Input: part model. Units: mm. Frame: model coordinates. Face numbers are marked on the shaded views. A direction names the side the tool comes from. Round coordinates to 2 decimals unless told otherwise and drop trailing zeros. Write each loop counter-clockwise with the first axis right and the second up, starting at its lowest first coordinate (ties: lowest second). Pieces come first, ordered by that corner, then holes. Notation, with made-up numbers: (56, -24) -> (60, -24) arc R15 cw to (60, -8) -> close; hole circle Ø7 at (66.5, -17.75). An arc over 180 degrees is marked (long way). Write item = value, one per line.
```python
from build123d import *

# Parameters (mm, degrees)
F0_W     = 58.7502
F0_H     = 43.18
F1_DEPTH = 22.225
F2_T     = -1.5875
F3_W     = 14.2875
F3_H     = 17.4625
F4_DEPTH = 3.175
F6_DEPTH = 0.79375
F7_R     = 2.54
F8_DEPTH = 6.35


with BuildPart() as f1:
    # F0 (on Front) → F1 (new body)
    with BuildSketch(Plane.XZ):
        with Locations((-10.3959683329, -10.1375534884)):
            Rectangle(F0_W, F0_H)
    extrude(amount=F1_DEPTH)

    # F2
    f2_openings = [f1.faces().sort_by_distance(p)[0] for p in [
        (-10.395968, -11.1125, 11.452447),
    ]]
    offset(amount=F2_T, openings=f2_openings)

    # F3 (on face) → F4 (cut)
    with BuildSketch(Plane.XZ.offset(22.225)):
        with BuildLine():
            Line((17.1960732201, 11.4524465116), (-11.3789267799, 11.4524465116))
            Line((-11.3789267799, 11.4524465116), (-11.3789267799, -3.0465692528))
            ThreePointArc((-11.3789267799, -3.0465692528), (2.9085732201, -13.7111715641), (17.1960732201, -3.0465692528))
            Line((17.1960732201, -3.0465692528), (17.1960732201, 11.4524465116))
        make_face()
        with Locations((-28.0476767799, -1.7169438296)):
            Rectangle(F3_W, F3_H)
        with BuildLine():
            Line((-13.4438804602, -15.5461690363), (-27.7313804602, -15.5461690363))
            ThreePointArc((-27.7313804602, -15.5461690363), (-34.0813804602, -21.8961690363), (-27.7313804602, -28.2461690363))
            Line((-27.7313804602, -28.2461690363), (-13.4438804602, -28.2461690363))
            Line((-13.4438804602, -28.2461690363), (-13.4438804602, -15.5461690363))
        make_face()
    extrude(amount=-F4_DEPTH, mode=Mode.SUBTRACT)

    # F5 (on face) → F6 (cut)
    with BuildSketch(Plane.YZ.offset(18.9791316671)):
        with BuildLine():
            ThreePointArc((-7.3954814436, -11.5285062603), (-7.2071898997, -10.8443275565), (-7.14375, -10.1375534884))
            ThreePointArc((-7.14375, -10.1375534884), (-7.1517294651, -9.8860115785), (-7.1756357738, -9.6354811558))
            Line((-7.1756357738, -9.6354811558), (-7.3954814436, -11.5285062603))
        make_face()
        with BuildLine():
            Line((-7.3954814436, -11.5285062603), (-7.1756357738, -9.6354811558))
            ThreePointArc((-7.1756357738, -9.6354811558), (-11.1125, -6.1688034884), (-15.0493642262, -9.6354811558))
            Line((-15.0493642262, -9.6354811558), (-14.8295185564, -11.5285062603))
            ThreePointArc((-14.8295185564, -11.5285062603), (-11.1125, -14.1063034884), (-7.3954814436, -11.5285062603))
        make_face()
        with BuildLine():
            ThreePointArc((-15.0493642262, -9.6354811558), (-11.1125, -6.1688034884), (-7.1756357738, -9.6354811558))
            Line((-7.1756357738, -9.6354811558), (-8.73125, 2.5624465116))
            ThreePointArc((-8.73125, 2.5624465116), (-11.1125, 0.1811965116), (-13.49375, 2.5624465116))
            Line((-13.49375, 2.5624465116), (-15.0493642262, -9.6354811558))
        make_face()
        with BuildLine():
            Line((-8.7408400071, -23.1129852184), (-7.3954814436, -11.5285062603))
            ThreePointArc((-7.3954814436, -11.5285062603), (-11.1125, -14.1063034884), (-14.8295185564, -11.5285062603))
            Line((-14.8295185564, -11.5285062603), (-13.4841599929, -23.1129852184))
            ThreePointArc((-13.4841599929, -23.1129852184), (-11.2504462955, -20.4539418213), (-8.7249, -22.8375534884))
            ThreePointArc((-8.7249, -22.8375534884), (-8.7288883329, -22.9754997838), (-8.7408400071, -23.1129852184))
        make_face()
        with BuildLine():
            Line((-14.8295185564, -11.5285062603), (-15.0493642262, -9.6354811558))
            ThreePointArc((-15.0493642262, -9.6354811558), (-15.0547539776, -10.5953854865), (-14.8295185564, -11.5285062603))
        make_face()
        with BuildLine():
            ThreePointArc((-13.49375, 2.5624465116), (-11.1125, 0.1811965116), (-8.73125, 2.5624465116))
            ThreePointArc((-8.73125, 2.5624465116), (-11.1125, 4.9436965116), (-13.49375, 2.5624465116))
        make_face()
        with BuildLine():
            ThreePointArc((-13.4841599929, -23.1129852184), (-11.1125, -25.2251534884), (-8.7408400071, -23.1129852184))
            ThreePointArc((-8.7408400071, -23.1129852184), (-8.7288883329, -22.9754997838), (-8.7249, -22.8375534884))
            ThreePointArc((-8.7249, -22.8375534884), (-11.2504462955, -20.4539418213), (-13.4841599929, -23.1129852184))
        make_face()
    extrude(amount=-F6_DEPTH, mode=Mode.SUBTRACT)

    # F7 (on face) → F8 (join)
    with BuildSketch(Plane(origin=(-39.7710683329, 0, 0), x_dir=(0, -1, 0), z_dir=(-1, 0, 0))):
        with Locations((11.1125, -10.1375534884)):
            Circle(F7_R)
    extrude(amount=F8_DEPTH)


solid = f1.part
```
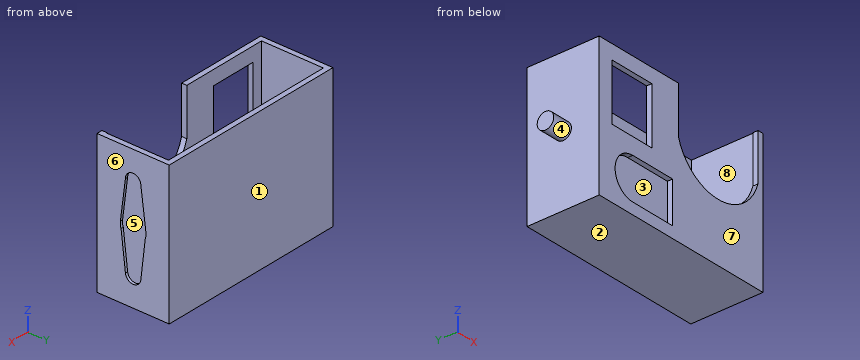
1) Cut plane B-B (y = -3.75). Return the cut outline in (x, z), and give its area (3 significant figures).
Solutions:
outline = (-39.77, -31.73) -> (18.98, -31.73) -> (18.98, 11.45) -> (17.39, 11.45) -> (17.39, -30.14) -> (-38.18, -30.14) -> (-38.18, 11.45) -> (-39.77, 11.45) -> close
area = 225 mm^2
2) Access query for the marked faces 1, 2, 3, 4 and 5. Directions: +Z, -Z, +X, -X, +Y, -Y. A direction counts if a zero-diameter tool reaches every point of the face in a straight line with its end or side. Return the directions, or none.
Solutions:
face_1 = +Z, -Z, +X, -X, +Y
face_2 = -Z, +X, -X, +Y, -Y
face_3 = +Z
face_4 = -X
face_5 = +X
3) Line query: L1, parallel to X at y = -15.5, z = -11; L2, parallel to Y at x = 11.5, z = -18.5 (1 decimal); L3, parallel to X at y = -11.75, z = -5. Output: solid intervals per line, ascending. Write a range as from..to.
Solutions:
L1 = -39.77..-38.18, 17.39..18.98
L2 = -22.2..-20.6, -1.6..0
L3 = -39.77..-38.18, 17.39..18.19
4) Cut plane C-C (z = -20.5). Return the cut outline in (x, y) (1 decimal).
Solutions:
outline = (-39.8, -22.2) -> (-33.9, -22.2) -> (-33.9, -20.6) -> (-38.2, -20.6) -> (-38.2, -1.6) -> (17.4, -1.6) -> (17.4, -20.6) -> (-13.4, -20.6) -> (-13.4, -22.2) -> (19, -22.2) -> (19, -13.8) -> (18.2, -13.8) -> (18.2, -8.4) -> (19, -8.4) -> (19, 0) -> (-39.8, 0) -> close
5) Draft query along Y for the marked faces 6, 7 and 8. Return one class per face: +Y half, -Y half, draft (parallel to the pull), parting line (faces both ways), or undercut.
Solutions:
face_6 = draft
face_7 = -Y half
face_8 = undercut
6) Cut plane A-A (x = -12.5). Return the cut outline in (y, z) (1 decimal).
Solutions:
outline = (-22.2, -31.7) -> (0, -31.7) -> (0, 11.5) -> (-1.6, 11.5) -> (-1.6, -30.1) -> (-20.6, -30.1) -> (-20.6, 11.5) -> (-22.2, 11.5) -> close
7) First-contact query: P1, Ø12, axis at y = -5, z = -2, coming from the -X side; P2, Ø5.5, axis at x = -1, y = -6.5, coming from the +Z side. Flat tips, straight axial feed; report the tip coordinate or a pass-through.
Solutions:
P1 = -39.77
P2 = -30.14
8) Cut plane D-D (y = -10.5). Return the cut outline in (x, z), and give its area (3 significant figures).
Solutions:
outline = (-46.12, -12.6) -> (-39.77, -12.6) -> (-39.77, -31.73) -> (18.98, -31.73) -> (18.98, -25.15) -> (18.19, -25.15) -> (18.19, 4.86) -> (18.98, 4.86) -> (18.98, 11.45) -> (17.39, 11.45) -> (17.39, -30.14) -> (-38.18, -30.14) -> (-38.18, 11.45) -> (-39.77, 11.45) -> (-39.77, -7.67) -> (-46.12, -7.67) -> close
area = 233 mm^2
